Model file for the job. Use its own axes, mm. A direction names the side the tool comes from. Round coordinates to 2 decimals unless told otherwise and drop trailing zeros. Loops run counter-clockwise (first coordinate to the right, second up) from the corner with the lowest first, then second, coordinate; pieces in that order, holes last. Notation, with made-up numbers: M -18.75,-1.5 L 11.25,-1.5 A16 cw 11.25,4.5 Z; hole C 47,25.5 d3. An arc over 180 degrees is marked long. Answer in a Markdown table with one row per item.
from build123d import *

# Parameters (mm, degrees)
EXTRUDE1_DEPTH          = 5.5
SKETCH2_R               = 1.6
SKETCH2_R_2             = 1.5
CUT_EXTRUDE1_DEPTH      = 20.5
CUT_EXTRUDE1_DEPTH_BACK = 19.5
CHAMFER1_SIZE           = 2
CHAMFER1_SIZE2          = 1.154700538
CHAMFER1_PART_2_SIZE    = 2
CHAMFER1_PART_2_SIZE2   = 1.154700538


with BuildPart() as part:
    # Sketch1 → Extrude1 (new body, symmetric)
    with BuildSketch(Plane.XY):
        with BuildLine():
            Line((61, -2), (61, -6.5))
            Line((61, -6.5), (11, -6.5))
            Line((11, -6.5), (11, -18.5))
            Line((11, -18.5), (-30, -18.5))
            Line((-30, -18.5), (-85, -4))
            Line((-85, -4), (-85, -3))
            Line((-85, -3), (-42.196152423, -3))
            ThreePointArc((-42.196152423, -3), (-31, 0), (-42.196152423, 3))
            Line((-42.196152423, 3), (-85, 3))
            Line((-85, 3), (-85, 4))
            Line((-85, 4), (-30, 18.5))
            Line((-30, 18.5), (11, 18.5))
            Line((11, 18.5), (11, 19.5))
            Line((11, 19.5), (61, 19.5))
            Line((61, 19.5), (61, 2))
            Line((61, 2), (48, 2))
            Line((48, 2), (48, -2))
            Line((48, -2), (61, -2))
        make_face()
    extrude(amount=EXTRUDE1_DEPTH, both=True)

    # Sketch2 → Cut-Extrude1 (cut, two sides)
    with BuildSketch(Plane(origin=(0, 0, 0), x_dir=(1, 0, 0), z_dir=(0, 1, 0))) as cut_extrude1_sk:
        with Locations(Location((21, 0, 0), (0, 0, 270))):  # turned: the seam where the file's is
            Circle(SKETCH2_R)
        with Locations(Location((51, 0, 0), (0, 0, 270))):  # turned: the seam where the file's is
            Circle(SKETCH2_R)
        with Locations((-63, 0)):
            Circle(SKETCH2_R_2)
    extrude(amount=CUT_EXTRUDE1_DEPTH, mode=Mode.SUBTRACT)
    extrude(cut_extrude1_sk.sketch, amount=-CUT_EXTRUDE1_DEPTH_BACK, mode=Mode.SUBTRACT)

    # Chamfer1
    chamfer1_edges = [part.edges().sort_by_distance(p)[0] for p in [
        (-63.598076211, -3, 5.5),
    ]]
    chamfer1_side = [part.faces().sort_by_distance(p)[0] for p in [
        (-63.598076211, -3, -5.058053242),
    ]]
    chamfer(chamfer1_edges, length=CHAMFER1_SIZE, length2=CHAMFER1_SIZE2, reference=chamfer1_side[0])

    # Chamfer1 part 2
    chamfer1_part_2_edges = [part.edges().sort_by_distance(p)[0] for p in [
        (-63.598076211, 3, 5.5),
    ]]
    chamfer1_part_2_side = [part.faces().sort_by_distance(p)[0] for p in [
        (-63.598076211, 3, -5.058053242),
    ]]
    chamfer(chamfer1_part_2_edges, length=CHAMFER1_PART_2_SIZE, length2=CHAMFER1_PART_2_SIZE2, reference=chamfer1_part_2_side[0])

    # Sketch3 → Cut-Revolve1 (revolve, cut)
    with BuildSketch(Plane(origin=(0, 0, 0), x_dir=(1, 0, 0), z_dir=(0, 1, 0))):
        Polygon((-10, 5.5), (-8.5, 5.5), (-8.5, 3.5), (2.5, 3.5), (2.5, -5.5), (-10, -5.5), align=None)
    revolve(axis=Axis((-10, 0, -5.5), (0, 0, -1)), mode=Mode.SUBTRACT)


solid = part.part
1. Pin check, flat tips, straight feed: pin 1 (20 mm diameter, centred on x = -10, y = 0, fed in from +Z); pin 2 (8 mm diameter, centred on x = 39.5, y = -14, fed in from +Z); pin 3 (3 mm diameter, centred on x = -8, z = 2, fed in from +Y); pin 4 (4 mm diameter, centred on x = 51, z = 0, fed in from -Y). Stop position of each tip, or through.
Verdict:
| item | result |
|---|---|
| pin 1 | stops at z = -3.5 |
| pin 2 | passes through |
| pin 3 | stops at y = 18.5 |
| pin 4 | stops at y = -6.5 |
2. Saw through at D-D (z = 0). State how many separate pieces and enclosed holes the cut face has, and give its area (3 significant figures).
Verdict:
| item | result |
|---|---|
| separate pieces | 6 |
| enclosed holes | 1 |
| area | 2,950 mm² |
3. Saw through at B-B (x = 21). Write the cut outline in (y, z).
Verdict:
| item | result |
|---|---|
| outline | M -6.5,-5.5 L 19.5,-5.5 L 19.5,-1.6 L -6.5,-1.6 Z; M -6.5,1.6 L 19.5,1.6 L 19.5,5.5 L -6.5,5.5 Z |
4. Tool access for faces 1 (the flat face through (48, 0, 0)), 2 (the flat face through (-64, -3, -2)), 3 (the flat face through (11, -12, 0)), 4 (the flat face through (-10, 3, -3.5)): list every direction of +Z, -Z, +X, -X, +Y, -Y with a clear straight run to the whole face (end or side of a thin tool).
Verdict:
| item | result |
|---|---|
| face 1 | +Z, -Z, +X |
| face 2 | +Z, -Z, -X |
| face 3 | +Z, -Z, +X, -Y |
| face 4 | +Z |
5. Saw through at A-A (y = 0). Write the cut outline in (x, z).
Verdict:
| item | result |
|---|---|
| outline | M -31,-5.5 L -11.5,-5.5 L -11.5,-3.5 L -22.5,-3.5 L -22.5,5.5 L -31,5.5 Z; M -8.5,-5.5 L 48,-5.5 L 48,5.5 L 2.5,5.5 L 2.5,-3.5 L -8.5,-3.5 Z; hole C 21,0 d3.2 |
6. Saw through at C-C (x = -63). Write the cut outline in (y, z).
Verdict:
| item | result |
|---|---|
| outline | M -9.8,-5.5 L -3,-5.5 L -3,-1.5 L -9.8,-1.5 Z; M -9.8,1.5 L -3,1.5 L -3,3.5 L -4.15,5.5 L -9.8,5.5 Z; M 3,-5.5 L 9.8,-5.5 L 9.8,-1.5 L 3,-1.5 Z; M 3,1.5 L 9.8,1.5 L 9.8,5.5 L 4.15,5.5 L 3,3.5 Z |
7. Mould opens along X. For faces 5 (the flat face through (61, 11, 0)), 6 (the cylindrical face through (-61.57, -6.55, -0.45)), 7 (the flat face through (54, -2, 0)) say: +X half, -X half, draft (parallel to the pull), parting line (faces both ways), or undercut.
Verdict:
| item | result |
|---|---|
| face 5 | +X half |
| face 6 | undercut |
| face 7 | draft |
8. Wall check: probe 1 along Y at (x, z) = (50, -3.25); probe 2 along X at (y, z) = (0, 0); probe 3 along X at (y, z) = (0, -1). Give the ranges that are in metal, low to high.
Verdict:
| item | result |
|---|---|
| probe 1 | y = -6.5 to -2, 2 to 19.5 |
| probe 2 | x = -31 to -22.5, 2.5 to 19.4, 22.6 to 48 |
| probe 3 | x = -31 to -22.5, 2.5 to 19.75, 22.25 to 48 |
